from build123d import *

# Parameters (mm, degrees)
F0_W     = 109.9
F0_H     = 91.3
F1_DEPTH = 2
F2_R     = 1.5
F3_DEPTH = 25.4
F4_W     = 25.296519
F4_H     = 16.046952
F5_DEPTH = 12.7
F6_W     = 7.949238
F6_H     = 62.397955
F7_DEPTH = 12.7
F8_W     = 7.973293
F8_H     = 72.191391
F8_W_2   = 76.933302
F8_H_2   = 27.90428
F9_DEPTH = 12.7


with BuildPart() as f1:
    # F0 (on Top) → F1 (new body)
    with BuildSketch(Plane.XY):
        with Locations((54.95, 45.65)):
            Rectangle(F0_W, F0_H)
    extrude(amount=F1_DEPTH)

    # F2 (on face) → F3 (cut)
    with BuildSketch(Plane.XY.offset(2)):
        with Locations((3.6, 88.5)):
            Circle(F2_R)
        with Locations((108.1, 3)):
            Circle(F2_R)
        with Locations((107.8, 89)):
            Circle(F2_R)
        with Locations((2.8, 3)):
            Circle(F2_R)
        with Locations((74.3, 54.1)):
            Circle(F2_R)
    extrude(amount=-F3_DEPTH, mode=Mode.SUBTRACT)

    # F4 (on face) → F5 (join)
    with BuildSketch(Plane.XY.offset(2)):
        with Locations((26.327649, 0.037087)):
            Rectangle(F4_W, F4_H)
    extrude(amount=F5_DEPTH)

    # F6 (on face) → F7 (join)
    with BuildSketch(Plane.XY.offset(2)):
        with Locations((7.164945, 50.75232)):
            Rectangle(F6_W, F6_H)
    extrude(amount=F7_DEPTH)

    # F8 (on face) → F9 (join)
    with BuildSketch(Plane.XY.offset(2)):
        with Locations((105.913353, 47.034552)):
            Rectangle(F8_W, F8_H)
        with Locations((54.388795, 73.369596)):
            Rectangle(F8_W_2, F8_H_2)
    extrude(amount=F9_DEPTH)


solid = f1.part
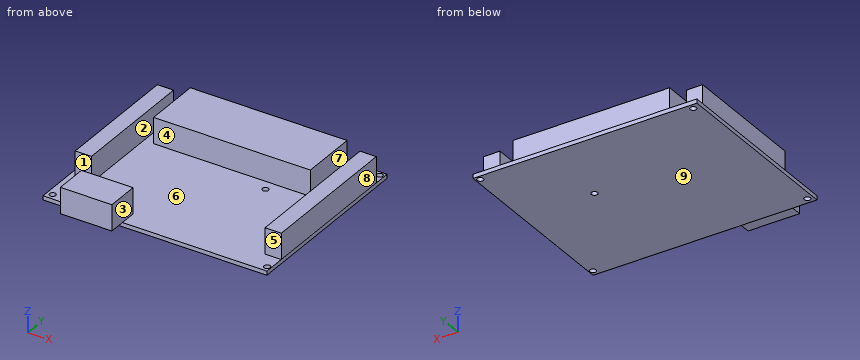
Source: CAD feature listing. Evaluate the final solid. Frame: model axes, mm. Face numbers are marked on the shaded views. A direction names the side the tool comes from. Round coordinates to 2 decimals unless told otherwise and drop trailing zeros. Loops run counter-clockwise (first coordinate to the right, second up) from the corner with the lowest first, then second, coordinate; pieces in that order, holes last. Notation, with made-up numbers: (62.5, -8) - (94.5, -8) arc R16 cw to (94.5, 5) - close; hole circle Ø4 at (34, 16). An arc over 180 degrees is marked (long way). Write item = value, one per line. Start each with the question number.
(1) Section query A-A, the plane z = 8. Output: boundary loops of the cut face in (x, y).
(2) Section query C-C, the plane x = 74.3. Output: boundary loops of the cut face in (y, z).
(3) Section query B-B, the plane y = 54.1. Output: boundary loops of the cut face in (x, z), plus the area to 3 significant figures.
(4) Ray query, line 1 along Y through (x, z) = (107.8, 1.45); line 2 along X through (y, z) = (28, 9); line 3 along X through (y, z) = (69, 9.25). Return the intervals inside material, ascending. Write a range as from..to.
(5) Pull-direction query (X, two-part tool) for the marked faces 6, 7, 8 and 9; classes: +X half, -X half, draft (parallel to the pull), parting line (faces both ways), or undercut.
(6) Set-up query: the marked faces 1, 2, 3, 4 and 5. Return all of +Z, -Z, +X, -X, +Y, -Y with unobstructed straight access to the full face (end or side cutting, diameter ignored); none if empty.
(7) Pin query (flat end, axial travel): pin 1 (6 mm diameter, centred on x = 73.5, y = 24.5, fed in from +Z); pin 2 (2.5 mm diameter, centred on x = 23.5, y = -2.5, fed in from -Z); pin 3 (6.5 mm diameter, centred on y = 79.5, z = 7, fed in from -X). Return the tip coordinate at first contact, or that it passes through.
(8) Section query D-D, the plane x = 53.5. Output: boundary loops of the cut face in (y, z), plus the area to 3 significant figures.
Conclusion:
q1.outline = (3.19, 19.55) - (11.14, 19.55) - (11.14, 81.95) - (3.19, 81.95) - close; (13.68, -7.99) - (38.98, -7.99) - (38.98, 8.06) - (13.68, 8.06) - close; (15.92, 59.42) - (92.86, 59.42) - (92.86, 87.32) - (15.92, 87.32) - close; (101.93, 10.94) - (109.9, 10.94) - (109.9, 83.13) - (101.93, 83.13) - close
q2.outline = (0, 0) - (52.6, 0) - (52.6, 2) - (0, 2) - close; (55.6, 0) - (91.3, 0) - (91.3, 2) - (87.32, 2) - (87.32, 14.7) - (59.42, 14.7) - (59.42, 2) - (55.6, 2) - close
q3.outline = (0, 0) - (72.8, 0) - (72.8, 2) - (11.14, 2) - (11.14, 14.7) - (3.19, 14.7) - (3.19, 2) - (0, 2) - close; (75.8, 0) - (109.9, 0) - (109.9, 14.7) - (101.93, 14.7) - (101.93, 2) - (75.8, 2) - close
q3.area = 416 mm2
q4.line_1 = 0..1.53, 4.47..87.5, 90.5..91.3
q4.line_2 = 3.19..11.14, 101.93..109.9
q4.line_3 = 3.19..11.14, 15.92..92.86, 101.93..109.9
q5.face_6 = undercut
q5.face_7 = undercut
q5.face_8 = +X half
q5.face_9 = draft
q6.face_1 = +Z, -X, -Y
q6.face_2 = +Z, +Y, -Y
q6.face_3 = +Z, +X, -Y
q6.face_4 = +Z
q6.face_5 = +Z, +X, -X, -Y
q7.pin_1 = 2
q7.pin_2 = 2
q7.pin_3 = 3.19
q8.outline = (0, 0) - (91.3, 0) - (91.3, 2) - (87.32, 2) - (87.32, 14.7) - (59.42, 14.7) - (59.42, 2) - (0, 2) - close
q8.area = 537 mm2
